For this review, take the finished solid that the model builds, in its own axes (mm). Face numbers are marked on the shaded views. A direction names the side the tool comes from. Give positions to 0.01 mm unless a question says otherwise; leave off trailing zeros. Loops run counter-clockwise (first coordinate to the right, second up) from the corner with the lowest first, then second, coordinate; pieces in that order, holes last. Notation, with made-up numbers: (27, 56.25) - (35, 56.25) arc R22 ccw to (35, 68.25) - close; hole circle Ø5 at (75.5, -17.5). An arc over 180 degrees is marked (long way). Answer as CSV lines item,"result".
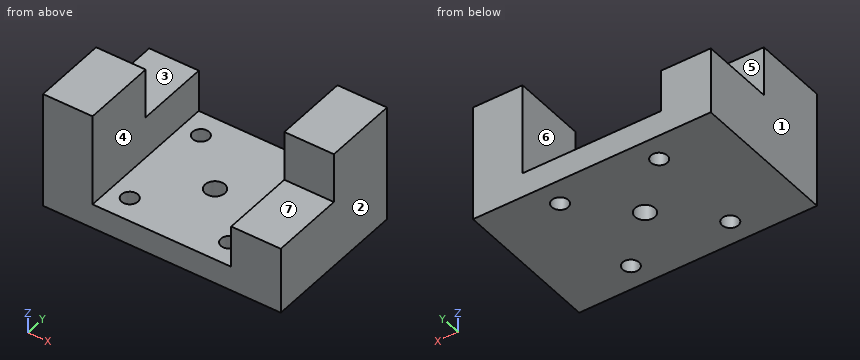
from build123d import *

# Parameters (mm, degrees)
SKETCH1_W           = 48
SKETCH1_H           = 30
SKETCH1_R           = 1.65
SKETCH1_R_2         = 2
BOSS_EXTRUDE1_DEPTH = 5
SKETCH2_W           = 10
SKETCH2_H           = 15
BOSS_EXTRUDE2_DEPTH = 18.61
SKETCH2_3_W         = 10
SKETCH2_3_H         = 15
BOSS_EXTRUDE3_DEPTH = 8.51


with BuildPart() as part:
    # Sketch1 → Boss-Extrude1 (new body)
    with BuildSketch(Plane.XY):
        Rectangle(SKETCH1_W, SKETCH1_H)
        with Locations((-10, 10)):
            Circle(SKETCH1_R, mode=Mode.SUBTRACT)
        with Locations((10, 10)):
            Circle(SKETCH1_R, mode=Mode.SUBTRACT)
        with Locations((10, -10)):
            Circle(SKETCH1_R, mode=Mode.SUBTRACT)
        with Locations((-9.995165444, -10.096450463)):
            Circle(SKETCH1_R, mode=Mode.SUBTRACT)
        Circle(SKETCH1_R_2, mode=Mode.SUBTRACT)
    extrude(amount=BOSS_EXTRUDE1_DEPTH)

    # Sketch2 → Boss-Extrude2 (add)
    with BuildSketch(Plane.XY.offset(5)):
        with Locations((19, 7.5)):
            Rectangle(SKETCH2_W, SKETCH2_H)
        with Locations((-19, -7.5)):
            Rectangle(SKETCH2_W, SKETCH2_H)
    extrude(amount=BOSS_EXTRUDE2_DEPTH)

    # Sketch2<3> → Boss-Extrude3 (add)
    with BuildSketch(Plane.XY.offset(5)):
        with Locations((19, -7.5)):
            Rectangle(SKETCH2_3_W, SKETCH2_3_H)
        with Locations((-19, 7.5)):
            Rectangle(SKETCH2_3_W, SKETCH2_3_H)
    extrude(amount=BOSS_EXTRUDE3_DEPTH)


solid = part.part
1) Consider section C-C on y = 7.75. Write out the cut boundary in (x, z), and give its area (3 significant figures).
From the geometry:
outline,"(-24, 0) - (24, 0) - (24, 23.61) - (14, 23.61) - (14, 5) - (-14, 5) - (-14, 13.51) - (-24, 13.51) - close"
area,"511 mm^2"
2) Consider section D-D on x = 10. Write out the cut boundary in (y, z), and give its area (3 significant figures).
From the geometry:
outline,"(-15, 0) - (-11.65, 0) - (-11.65, 5) - (-15, 5) - close; (-8.35, 0) - (8.35, 0) - (8.35, 5) - (-8.35, 5) - close; (11.65, 0) - (15, 0) - (15, 5) - (11.65, 5) - close"
area,"117 mm^2"
3) Machinability: for the marked faces 5, 6 and 7, which of the approach directions +Z, -Z, +X, -X, +Y, -Y give a long, thin tool a straight path to every point of the face, cutting with its end or side? Answer none if there is none.
From the geometry:
face 5,"+Z, -X, +Y"
face 6,"+Z, +Y, -Y"
face 7,"+Z, +X, -Y"
4) Draft analysis for pull direction X (two halves, no side actions). For the marked faces 1, 2, 3 and 4, state which applies: pulls with the +X half, pulls with the -X half, needs draft (parallel to the pull), parting line crosses it, or undercut.
From the geometry:
face 1,"pulls with the -X half"
face 2,"pulls with the +X half"
face 3,"needs draft"
face 4,"undercut"
5) Insertion check: P1, Ø11, axis at x = -18, z = 20.5, coming from the +Y side; P2, Ø14, axis at x = 6.5, y = -2, coming from the +Z side; P3, Ø3, axis at x = -17, y = 6, coming from the +Z side. Each pin has a flat end and moves straight along its axis. Give the tip position at first contact, or say it passes through.
From the geometry:
P1,"stops at y = 0"
P2,"stops at z = 5"
P3,"stops at z = 13.51"
6) Wall thickness on line 1 (Y direction, x = -10, z = 2); line 2 (Y direction, x = 10, z = 3.45); line 3 (Y direction, x = 0, z = 2.8): over which ranges is each line inside the solid? List them lowest first. Write a range as from..to.
From the geometry:
line 1,"y = -15..-11.75, -8.45..8.35, 11.65..15"
line 2,"y = -15..-11.65, -8.35..8.35, 11.65..15"
line 3,"y = -15..-2, 2..15"
7) Consider section B-B on x = 0. Write out the cut boundary in (y, z).
From the geometry:
outline,"(-15, 0) - (-2, 0) - (-2, 5) - (-15, 5) - close; (2, 0) - (15, 0) - (15, 5) - (2, 5) - close"
8) Consider section A-A on z = 12.5. Write out the cut boundary in (x, y), and give its area (3 significant figures).
From the geometry:
outline,"(-24, -15) - (-14, -15) - (-14, 15) - (-24, 15) - close; (14, -15) - (24, -15) - (24, 15) - (14, 15) - close"
area,"600 mm^2"
